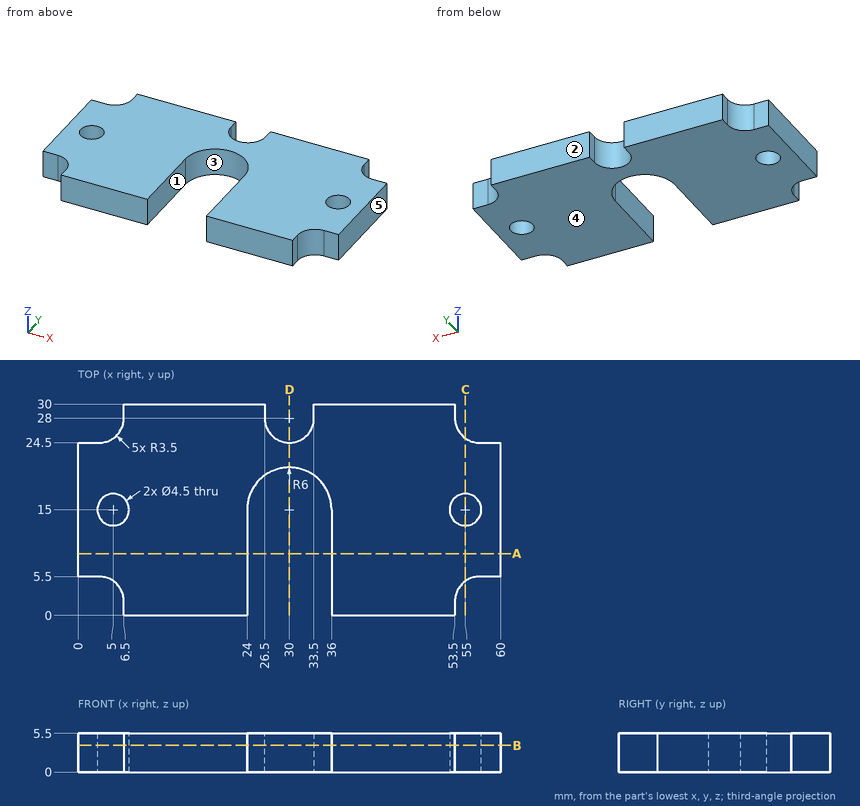
Input: dimensioned drawing with shaded views. Units: mm. Origin: part minimum x, y, z. A direction names the side the tool comes from. Give positions to 0.01 mm unless a question says otherwise; leave off trailing zeros. Write each loop counter-clockwise with the first axis right and the second up, starting at its lowest first coordinate (ties: lowest second). Pieces come first, ordered by that corner, then holes.
Q1. Section A-A, the plane y = 8.75. Output: boundary loops of the cut face in (x, z), plus the area to 3 significant figures.
Q2. Pull-direction query (X, two-part tool) for the marked faces 3, 4 and 5; classes: pulls with the +X half, pulls with the -X half, needs draft (parallel to the pull), parting line crosses it, or undercut.
Q3. Section D-D, the plane x = 30. Output: boundary loops of the cut face in (y, z).
Q4. First-contact query: P1, Ø1, axis at y = 29.5, z = 1.5, coming from the -X side; P2, Ø1.6, axis at y = 29.5, z = 4, coming from the +X side; P3, Ø2.5, axis at x = 58, z = 4, coming from the -Y side. Flat tips, straight axial feed; report the tip coordinate or a pass-through.
Q5. Section C-C, the plane x = 55. Output: boundary loops of the cut face in (y, z).
Q6. Section B-B, the plane z = 3.8. Output: boundary loops of the cut face in (x, y).
Q7. Material intervals for probe 1 along X at (y, z) = (15.75, 4.05); probe 2 along X at (y, z) = (17, 1.15); probe 3 along Y at (x, z) = (5, 3.65), sorted ascending.
Q8. Set-up query: the marked faces 1 and 2. Return all of +Z, -Z, +X, -X, +Y, -Y with unobstructed straight access to the full face (end or side cutting, diameter ignored); none if empty.
Filled in:
1. outline: (0, 0) - (24, 0) - (24, 5.5) - (0, 5.5) - close; (36, 0) - (60, 0) - (60, 5.5) - (36, 5.5) - close
1. area: 264 mm2
2. face 3: undercut
2. face 4: needs draft
2. face 5: pulls with the +X half
3. outline: (21, 0) - (24.5, 0) - (24.5, 5.5) - (21, 5.5) - close
4. P1: stops at x = 6.5
4. P2: stops at x = 53.5
4. P3: stops at y = 5.49
5. outline: (4.87, 0) - (12.75, 0) - (12.75, 5.5) - (4.87, 5.5) - close; (17.25, 0) - (25.13, 0) - (25.13, 5.5) - (17.25, 5.5) - close
6. outline: (0, 5.5) - (3, 5.5) arc R3.5 cw to (6.5, 2) - (6.5, 0) - (24, 0) - (24, 15) arc R6 cw to (36, 15) - (36, 0) - (53.5, 0) - (53.5, 2) arc R3.5 cw to (57, 5.5) - (60, 5.5) - (60, 24.5) - (57, 24.5) arc R3.5 cw to (53.5, 28) - (53.5, 30) - (33.5, 30) - (33.5, 28) arc R3.5 cw to (26.5, 28) - (26.5, 30) - (6.5, 30) - (6.5, 28) arc R3.5 cw to (3, 24.5) - (0, 24.5) - close; hole circle Ø4.5 at (5, 15); hole circle Ø4.5 at (55, 15)
7. probe 1: x = 0 to 2.88, 7.12 to 24.05, 35.95 to 52.88, 57.12 to 60
7. probe 2: x = 0 to 3.97, 6.03 to 24.34, 35.66 to 53.97, 56.03 to 60
7. probe 3: y = 4.87 to 12.75, 17.25 to 25.13
8. face 1: +Z, -Z, -Y
8. face 2: +Z, -Z, +X, -X, +Y
